Source: three-view drawing plus pictorial views. Frame: mm from the lowest corner of the part. A direction names the side the tool comes from. Round coordinates to 2 decimals unless told otherwise and drop trailing zeros. Order: outer loops, then holes, each group sorted by start corner. A loop starts at its lowest first (then second) coordinate and runs counter-clockwise, first axis right, second up. Notation, with made-up numbers: M -15,13 L 14,13 A21 cw 14,17 Z; hole C 47,-3.5 d2. An arc over 180 degrees is marked long. Return JSON: item names as keys, results as strings. Group by question number.
Q1. Cut plane D-D on x = 20. Output: boundary loops of the cut face in (y, z) (1 decimal).
Q2. Cut plane B-B on x = 13. Output: boundary loops of the cut face in (y, z).
Q3. Contact query for flat-ended pins moving along their axis: pin 1 (8 mm diameter, centred on x = 4, z = 19, fed in from -Y); pin 2 (3 mm diameter, centred on x = 16.5, y = 4, fed in from +Z); pin 3 (0.8 mm diameter, centred on y = 14, z = 16, fed in from -X); pin 4 (1 mm diameter, centred on x = 16.5, y = 12, fed in from +Z) (1 decimal). Output: stop coordinate, or through.
Q4. Ray query, probe 1 along X at (y, z) = (14.4, 32.5); probe 2 along Y at (x, z) = (4, 0.4) (1 decimal); probe 3 along Y at (x, z) = (13, 0.4) (1 decimal). Return the intervals inside material, ascending.
Q5. Cut plane A-A on y = 7.5. Output: boundary loops of the cut face in (x, z).
Q6. Access query for the marked faces 1 and 2. Directions: +Z, -Z, +X, -X, +Y, -Y. A direction counts if a zero-diameter tool reaches every point of the face in a straight line with its end or side. Return the directions, or none.
Q7. Cut plane C-C on z = 13.5. Output: boundary loops of the cut face in (x, y), and give its area (3 significant figures).
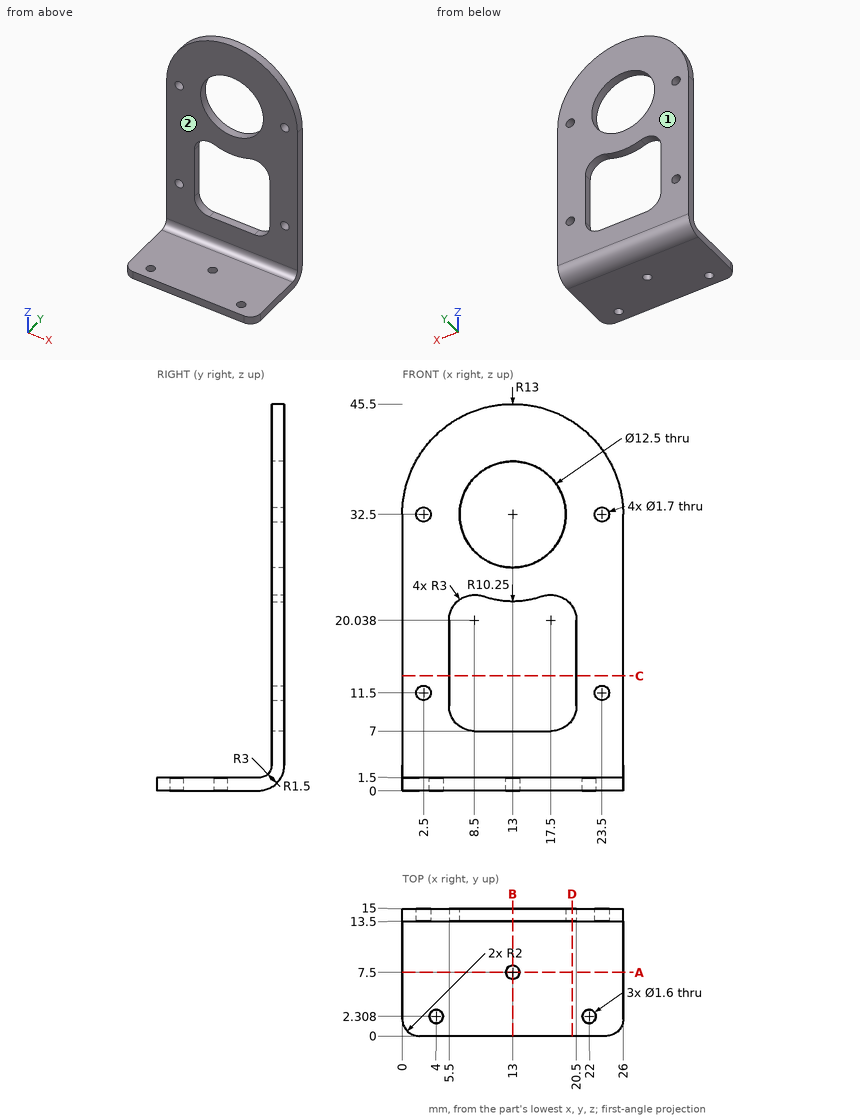
Result sheet:
{
 "1": {"outline": "M 0,0 L 12,0 A3 ccw 15,3 L 15,8.3 L 13.5,8.3 L 13.5,3 A1.5 cw 12,1.5 L 0,1.5 Z; M 13.5,21.7 L 15,21.7 L 15,43.5 L 13.5,43.5 Z"},
 "2": {"outline": "M 0,0 L 6.7,0 L 6.7,1.5 L 0,1.5 Z; M 8.3,0 L 12,0 A3 ccw 15,3 L 15,7 L 13.5,7 L 13.5,3 A1.5 cw 12,1.5 L 8.3,1.5 Z; M 13.5,22.25 L 15,22.25 L 15,26.25 L 13.5,26.25 Z; M 13.5,38.75 L 15,38.75 L 15,45.5 L 13.5,45.5 Z"},
 "3": {"pin 1": "stops at y = 13.5", "pin 2": "stops at z = 1.5", "pin 3": "stops at x = 0", "pin 4": "stops at z = 1.6"},
 "4": {"probe 1": "x = 0 to 1.65, 3.35 to 6.75, 19.25 to 22.65, 24.35 to 26", "probe 2": "y = 0 to 1.5, 3.1 to 13.5", "probe 3": "y = 0 to 6.7, 8.3 to 13.5"},
 "5": {"outline": "M 0,0 L 12.2,0 L 12.2,1.5 L 0,1.5 Z; M 13.8,0 L 26,0 L 26,1.5 L 13.8,1.5 Z"},
 "6": {"face 1": "+Z, -Z, +X, -X, +Y", "face 2": "+Z, +X, -X, -Y"},
 "7": {"outline": "M 0,13.5 L 5.5,13.5 L 5.5,15 L 0,15 Z; M 20.5,13.5 L 26,13.5 L 26,15 L 20.5,15 Z", "area": "16.5 mm²"}
}
